Input: part model. Units: mm. Frame: model coordinates. Face numbers are marked on the shaded views. A direction names the side the tool comes from. Give positions to 0.01 mm unless a question says otherwise; leave off trailing zeros. Loops run counter-clockwise (first coordinate to the right, second up) from the corner with the lowest first, then second, coordinate; pieces in that order, holes last. Notation, with made-up numbers: (-23, -26) - (24, -26) arc R20 cw to (24, -7) - close; hole circle Ø4 at (19, -9.75). An arc over 180 degrees is marked (long way). Answer as a JSON object with one key per item and string values.
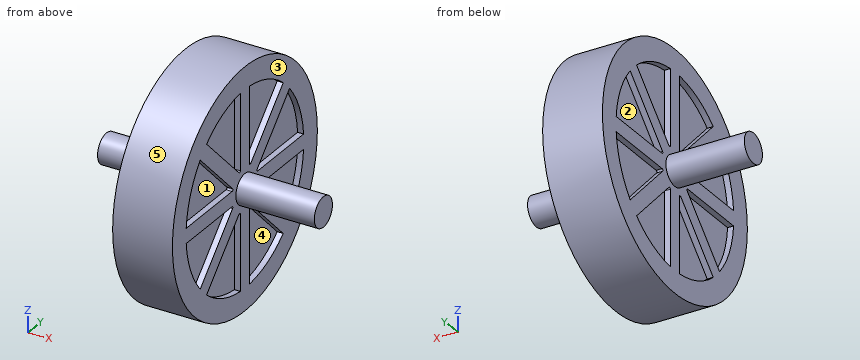
Autodesk Inventor part; units mm, degrees
ref_plane "YZ Plane" through (0, 0, 0) normal (1, 0, 0) x (0, 1, 0)
ref_plane "XZ Plane" through (0, 0, 0) normal (0, 1, 0) x (-1, 0, 0)
ref_plane "XY Plane" through (0, 0, 0) normal (0, 0, 1) x (1, 0, 0)
sketch "Sketch1" plane through (0, 0, 0) normal (1, 0, 0) x (0, 1, 0)
  circle A0 centre (0, 0) radius 50.8
  dimension "d0" = 101.6
extrude "Extrusion1" add sketch "Sketch1" along normal blind 25.4
sketch "Sketch2" plane through (25.4, 0, 0) normal (1, 0, 0) x (0, 0, -1)
  circle A0 centre (0, 0) radius 6.35
  dimension "d4" = 12.7
extrude "Extrusion2" add sketch "Sketch2" along normal blind 33.3375
sketch "Sketch3" plane through (0, 0, 0) normal (-1, 0, 0) x (0, 0, 1)
  circle A0 centre (0, 0) radius 6.35
extrude "Extrusion3" add sketch "Sketch3" along normal blind 33.3375
sketch "Sketch5" plane through (25.4, 0, 0) normal (1, 0, 0) x (0, 0, -1)
  circle A0 centre (0, 0) radius 44.45
  arc A1 (31.3429, -26.8561) -> (41.1529, -3.1727) centre (0, 0) ccw
  line L0 (0, 0) -> (82.55, 0) construction
  line L1 (41.1529, -3.1727) -> (8.9811, -3.1727)
  line L2 (31.3429, -26.8561) -> (82.1429, -26.8561) construction
  line L3 (31.3429, -26.8561) -> (8.594, -4.1072)
  line L4 (-4.1072, 8.594) -> (-4.5781, 9.0649)
  arc A2 (8.9811, -3.1727) -> (8.594, -4.1072) centre (8.9811, -3.7201) ccw
  arc A3 (41.1529, 3.1727) -> (31.3429, 26.8561) centre (0, 0) ccw
  line L5 (31.3429, 26.8561) -> (8.594, 4.1072)
  line L6 (41.1529, 3.1727) -> (8.9811, 3.1727)
  arc A4 (8.594, 4.1072) -> (8.9811, 3.1727) centre (8.9811, 3.7201) ccw
  arc A5 (26.8561, 31.3429) -> (3.1727, 41.1529) centre (0, 0) ccw
  line L7 (3.1727, 41.1529) -> (3.1727, 8.9811)
  line L8 (26.8561, 31.3429) -> (4.1072, 8.594)
  arc A6 (3.1727, 8.9811) -> (4.1072, 8.594) centre (3.7201, 8.9811) ccw
  arc A7 (-3.1727, 41.1529) -> (-26.8561, 31.3429) centre (0, 0) ccw
  line L9 (-26.8561, 31.3429) -> (-4.1072, 8.594)
  line L10 (-3.1727, 41.1529) -> (-3.1727, 8.9811)
  arc A8 (-4.1072, 8.594) -> (-3.1727, 8.9811) centre (-3.7201, 8.9811) ccw
  arc A9 (-31.3429, 26.8561) -> (-41.1529, 3.1727) centre (0, 0) ccw
  line L11 (-41.1529, 3.1727) -> (-8.9811, 3.1727)
  line L12 (-31.3429, 26.8561) -> (-8.594, 4.1072)
  arc A10 (-8.9811, 3.1727) -> (-8.594, 4.1072) centre (-8.9811, 3.7201) ccw
  arc A11 (-41.1529, -3.1727) -> (-31.3429, -26.8561) centre (0, 0) ccw
  line L13 (-31.3429, -26.8561) -> (-8.594, -4.1072)
  line L14 (-41.1529, -3.1727) -> (-8.9811, -3.1727)
  arc A12 (-8.594, -4.1072) -> (-8.9811, -3.1727) centre (-8.9811, -3.7201) ccw
  arc A13 (-26.8561, -31.3429) -> (-3.1727, -41.1529) centre (0, 0) ccw
  line L15 (-3.1727, -41.1529) -> (-3.1727, -8.9811)
  line L16 (-26.8561, -31.3429) -> (-4.1072, -8.594)
  arc A14 (-3.1727, -8.9811) -> (-4.1072, -8.594) centre (-3.7201, -8.9811) ccw
  arc A15 (3.1727, -41.1529) -> (26.8561, -31.3429) centre (0, 0) ccw
  line L17 (26.8561, -31.3429) -> (4.1072, -8.594)
  line L18 (3.1727, -41.1529) -> (3.1727, -8.9811)
  arc A16 (4.1072, -8.594) -> (3.1727, -8.9811) centre (3.7201, -8.9811) ccw
  dimension "d12" = 88.9
  dimension "d13" = 82.55
  dimension "d24" = 360
extrude "Extrusion5" cut sketch "Sketch5" against normal blind 2.54 contours L3 A2 L1 A1 | L4 L9 A7 L10 A8 | L6 A4 L5 A3 | L8 A6 L7 A5 | L12 A10 L11 A9 | L14 A12 L13 A11 | L16 A14 L15 A13 | L18 A16 L17 A15
sketch "Sketch6" plane through (0, 0, 0) normal (-1, 0, 0) x (0, 0, 1)
  circle A0 centre (0, 0) radius 44.45
  arc A1 (-31.3429, 26.8561) -> (-41.1529, 3.1727) centre (0, 0) ccw
  line L0 (-8.594, 4.1072) -> (-31.3429, 26.8561)
  line L1 (-41.1529, 3.1727) -> (-8.9811, 3.1727)
  line L2 (-41.1529, 3.1727) -> (-8.9811, 3.1727)
  line L3 (-8.594, 4.1072) -> (-31.3429, 26.8561)
  arc A2 (-8.9811, 3.1727) -> (-8.594, 4.1072) centre (-8.9811, 3.7201) ccw
  arc A3 (-41.1529, -3.1727) -> (-31.3429, -26.8561) centre (0, 0) ccw
  line L4 (-31.3429, -26.8561) -> (-8.594, -4.1072)
  line L5 (-8.9811, -3.1727) -> (-41.1529, -3.1727)
  arc A4 (-8.594, -4.1072) -> (-8.9811, -3.1727) centre (-8.9811, -3.7201) ccw
  arc A5 (-26.8561, -31.3429) -> (-3.1727, -41.1529) centre (0, 0) ccw
  line L6 (-3.1727, -41.1529) -> (-3.1727, -8.9811)
  line L7 (-4.1072, -8.594) -> (-26.8561, -31.3429)
  arc A6 (-3.1727, -8.9811) -> (-4.1072, -8.594) centre (-3.7201, -8.9811) ccw
  arc A7 (3.1727, -41.1529) -> (26.8561, -31.3429) centre (0, 0) ccw
  line L8 (26.8561, -31.3429) -> (4.1072, -8.594)
  line L9 (3.1727, -8.9811) -> (3.1727, -41.1529)
  arc A8 (4.1072, -8.594) -> (3.1727, -8.9811) centre (3.7201, -8.9811) ccw
  arc A9 (31.3429, -26.8561) -> (41.1529, -3.1727) centre (0, 0) ccw
  line L10 (41.1529, -3.1727) -> (8.9811, -3.1727)
  line L11 (8.594, -4.1072) -> (31.3429, -26.8561)
  arc A10 (8.9811, -3.1727) -> (8.594, -4.1072) centre (8.9811, -3.7201) ccw
  arc A11 (41.1529, 3.1727) -> (31.3429, 26.8561) centre (0, 0) ccw
  line L12 (31.3429, 26.8561) -> (8.594, 4.1072)
  line L13 (8.9811, 3.1727) -> (41.1529, 3.1727)
  arc A12 (8.594, 4.1072) -> (8.9811, 3.1727) centre (8.9811, 3.7201) ccw
  arc A13 (26.8561, 31.3429) -> (3.1727, 41.1529) centre (0, 0) ccw
  line L14 (3.1727, 41.1529) -> (3.1727, 8.9811)
  line L15 (4.1072, 8.594) -> (26.8561, 31.3429)
  arc A14 (3.1727, 8.9811) -> (4.1072, 8.594) centre (3.7201, 8.9811) ccw
  arc A15 (-3.1727, 41.1529) -> (-26.8561, 31.3429) centre (0, 0) ccw
  line L16 (-26.8561, 31.3429) -> (-4.1072, 8.594)
  line L17 (-3.1727, 8.9811) -> (-3.1727, 41.1529)
  arc A16 (-4.1072, 8.594) -> (-3.1727, 8.9811) centre (-3.7201, 8.9811) ccw
  dimension "d28" = 88.9
  dimension "d32" = 360
extrude "Extrusion6" cut sketch "Sketch6" against normal blind 2.54 contours L0 A2 L1 A1 | L5 A4 L4 A3 | L7 A6 L6 A5 | L9 A8 L8 A7 | L11 A10 L10 A9 | L13 A12 L12 A11 | L15 A14 L14 A13 | L17 A16 L16 A15
properties part number "Wheel"
Item 1: Cut plane C-C (x = 35). Return loops of the section in (y, z).
Geometry check:
{"outline": "circle Ø12.7 at (0, 0)"}
Item 2: Cut plane D-D (y = -36.5). Return loops of the section in (x, z), then the cut area to 3 significant figures.
Geometry check:
{"outline": "(0, -35.33) - (25.4, -35.33) - (25.4, -19.27) - (22.86, -19.27) - (22.86, -3.17) - (25.4, -3.17) - (25.4, 3.17) - (22.86, 3.17) - (22.86, 19.27) - (25.4, 19.27) - (25.4, 35.33) - (0, 35.33) - (0, 19.27) - (2.54, 19.27) - (2.54, 3.17) - (0, 3.17) - (0, -3.17) - (2.54, -3.17) - (2.54, -19.27) - (0, -19.27) - close", "area": "1,630 mm2"}
Item 3: Access query for the marked faces 1 and 2. Directions: +Z, -Z, +X, -X, +Y, -Y. A direction counts if a zero-diameter tool reaches every point of the face in a straight line with its end or side. Return the directions, or none.
Geometry check:
{"face 1": "+X", "face 2": "-X"}
Item 4: Cut plane A-A (y = 0). Return loops of the section in (x, z).
Geometry check:
{"outline": "(-33.34, -6.35) - (0, -6.35) - (0, -50.8) - (25.4, -50.8) - (25.4, -6.35) - (58.74, -6.35) - (58.74, 6.35) - (25.4, 6.35) - (25.4, 50.8) - (0, 50.8) - (0, 6.35) - (-33.34, 6.35) - close"}
Item 5: Mould query, pull axis Y, two halves, no side actions, for the marked faces 3, 4 and 5. Classes: released by +Y, released by -Y, zero draft, split by the parting line, or undercut.
Geometry check:
{"face 3": "zero draft", "face 4": "undercut", "face 5": "split by the parting line"}
Item 6: Material intervals for line 1 (Z direction, x = 2, y = -33); line 2 (X direction, y = 38, z = -9); line 3 (Y direction, x = 0.5, z = 34.5), sorted ascending. Write a range as [from, to].
Geometry check:
{"line 1": "z = [-38.62, -24.79], [-3.17, 3.17], [24.79, 38.62]", "line 2": "x = [2.54, 22.86]", "line 3": "y = [-37.29, -22.66], [-3.17, 3.17], [22.66, 37.29]"}
Item 7: Contact query for flat-ended pins moving along their axis: P1, Ø19, axis at y = -11, z = -18.5, coming from the +X side; P2, Ø1.3, axis at x = 23.5, y = -26.5, coming from the -Z side; P3, Ø19, axis at y = -15, z = -32, coming from the -X side. Output: stop coordinate, or through.
Geometry check:
{"P1": "stops at x = 25.4", "P2": "stops at z = -43.73", "P3": "stops at x = 0"}
